Job drawing, mm, ordinate dimensions from the low corner. One solid piece. Round coordinates to 2 decimals unless told otherwise and drop trailing zeros. Write each loop counter-clockwise with the first axis right and the second up, starting at its lowest first coordinate (ties: lowest second). Pieces come first, ordered by that corner, then holes.
1) Saw through at B-B (z = 31.75). Write the cut outline in (x, y), plus the area to 3 significant figures.
2) Flat gauge pin, fed straight in: pin 1 (12.5 mm diameter, centred on x = 427.57, z = 107.95, fed in from -Y). Where does the tip first touch, or does it go through?
3) Saw through at C-C (x = 76.2). Write the cut outline in (y, z).
4) Saw through at A-A (y = 2). State how many separate pieces and enclosed holes the cut face has, plus the area to 3 significant figures.
5) Wall check: probe 1 along Z at (x, y) = (38.1, 4); probe 2 along Z at (x, y) = (76.2, 2.5); probe 3 along Z at (x, y) = (488, 5.5). Give the ranges that are in metal, low to high.
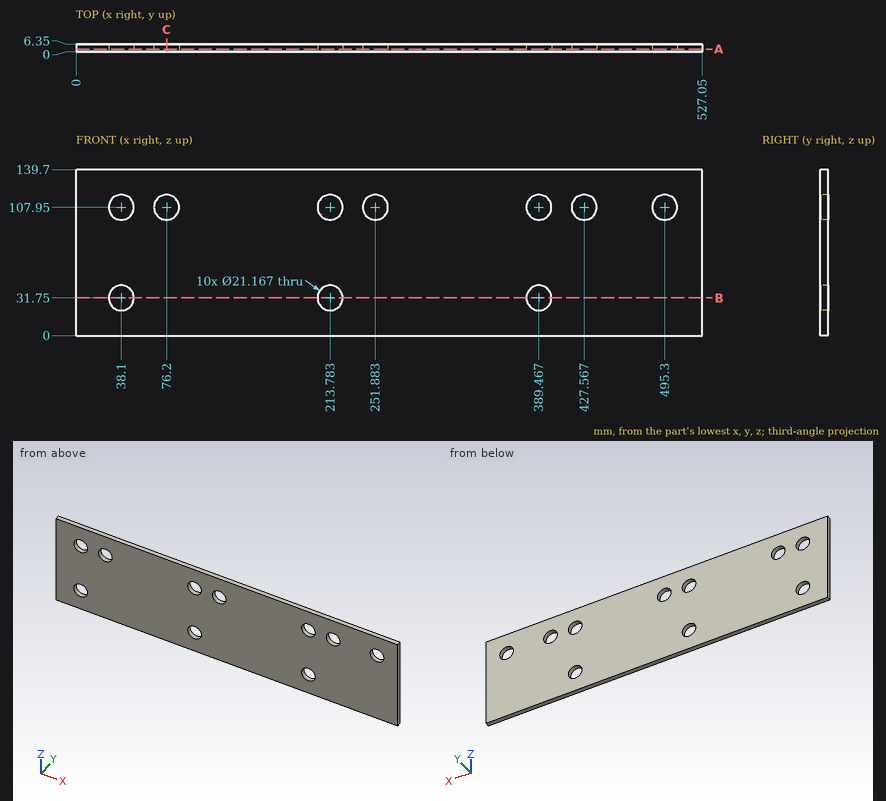
Evaluation:
1. outline: (0, 0) - (27.52, 0) - (27.52, 6.35) - (0, 6.35) - close; (48.68, 0) - (203.2, 0) - (203.2, 6.35) - (48.68, 6.35) - close; (224.37, 0) - (378.88, 0) - (378.88, 6.35) - (224.37, 6.35) - close; (400.05, 0) - (527.05, 0) - (527.05, 6.35) - (400.05, 6.35) - close
1. area: 2,940 mm2
2. pin 1: passes through
3. outline: (0, 0) - (6.35, 0) - (6.35, 97.37) - (0, 97.37) - close; (0, 118.53) - (6.35, 118.53) - (6.35, 139.7) - (0, 139.7) - close
4. separate pieces: 1
4. enclosed holes: 10
4. area: 70,100 mm2
5. probe 1: z = 0 to 21.17, 42.33 to 97.37, 118.53 to 139.7
5. probe 2: z = 0 to 97.37, 118.53 to 139.7
5. probe 3: z = 0 to 100.29, 115.61 to 139.7
